Check sheet for the drawn part. Datum: minimum x, y, z corner. Units: mm. A direction names the side the tool comes from. Coordinates: 2 decimals unless noted, no trailing zeros. Order: outer loops, then holes, each group sorted by start corner. A loop starts at its lowest first (then second) coordinate and runs counter-clockwise, first axis right, second up.
Q1. Draft check along Z on the marked faces 1 and 2. Enter one of: pulls with the +Z half, pulls with the -Z half, needs draft (parallel to the pull), parting line crosses it, or undercut.
Q2. Thickness scan on line 1 (X direction, y = 6.75, z = 15); line 2 (Z direction, x = 6.5, y = 4); line 3 (X direction, y = 1.5, z = 8). Record the ranges inside material, lowest first.
Q3. Cross-section at A-A, the plane z = 20. Record the boundary of the cut face in (x, y).
Q4. Depth check by flat-ended pin: P1, Ø3, axis at y = 5.5, z = 6.5, coming from the -X side; P2, Ø10, axis at x = 15.5, z = 17, coming from the +Y side; P3, Ø1, axis at x = 4, y = 4.5, coming from the +Z side. Enter the tip coordinate at first touch or a pass-through.
Q5. Cross-section at D-D, the plane x = 29.5. Record the boundary of the cut face in (y, z).
Q6. Set-up check for the marked faces 3 and 4: record each of +Z, -Z, +X, -X, +Y, -Y from which the full face is reachable in a straight line by a thin tool's end or side.
Q7. Cross-section at C-C, the plane z = 15. Record the boundary of the cut face in (x, y), and give its area (3 significant figures).
Q8. Cross-section at B-B, the plane y = 6.5. Record the boundary of the cut face in (x, z).
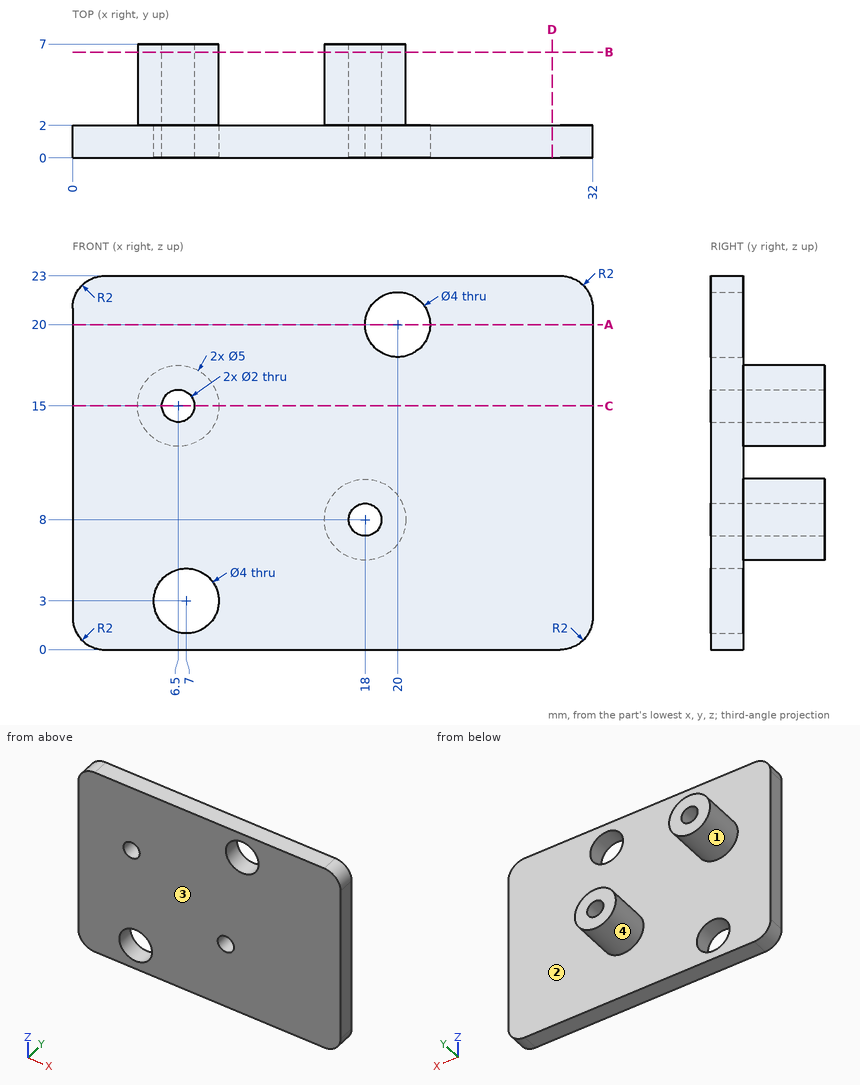
Check values:
1. face 1: parting line crosses it
1. face 2: needs draft
2. line 1: x = 4 to 5.5, 7.5 to 9
2. line 2: z = 12.5 to 14, 16 to 17.5
2. line 3: x = 0 to 17, 19 to 32
3. outline: (0, 0) - (18, 0) - (18, 2) - (0, 2) - close; (22, 0) - (32, 0) - (32, 2) - (22, 2) - close
4. P1: stops at x = 15.5
4. P2: stops at y = 2
4. P3: stops at z = 16.5
5. outline: (0, 0) - (2, 0) - (2, 23) - (0, 23) - close
6. face 3: +Z, -Z, +X, -X, -Y
6. face 4: +Y
7. outline: (0, 0) - (5.5, 0) - (5.5, 7) - (4, 7) - (4, 2) - (0, 2) - close; (7.5, 0) - (32, 0) - (32, 2) - (9, 2) - (9, 7) - (7.5, 7) - close
7. area: 75.0 mm2
8. outline: circle Ø5 at (6.5, 15); circle Ø5 at (18, 8); hole circle Ø2 at (6.5, 15); hole circle Ø2 at (18, 8)
